The listing builds one solid part. Answer for the finished solid, in the listing's coordinates (mm). Face numbers are marked on the shaded views. A direction names the side the tool comes from. Round coordinates to 2 decimals unless told otherwise and drop trailing zeros. Order: outer loops, then holes, each group sorted by start corner. A loop starts at its lowest first (then second) coordinate and runs counter-clockwise, first axis right, second up. Notation, with made-up numbers: (38.5, -37) - (87.5, -37) arc R15 cw to (87.5, -18) - close; hole circle Ø8 at (10.5, 62). An arc over 180 degrees is marked (long way). Use CSV: the item, a comma, the result in double quotes. Start each with the question number.
Item 1: Straight lines are drawn through the part: line 1 along Y through (x, z) = (-11, 1.75); line 2 along Y through (x, z) = (-7, 3.95); line 3 along Y through (x, z) = (12, 0.8). For each, find the intervals that lie inside material, in ascending order. Write a range as [from, to].
Item 2: Find section A-A, the plane x = -5.5. Give the vertices of the cut face in (y, z).
Item 3: Find section D-D, the plane y = -3.5. Give the vertices of the cut face in (x, z), plus the area to 3 significant figures.
Item 4: Find section B-B, the plane z = 3.1. Count the separate pieces of the cut face and the enclosed holes in it, plus the area to 3 significant figures.
Item 5: For the marked faces 1 and 2, determine the directions among +Z, -Z, +X, -X, +Y, -Y from which every point of the face is accessible in a straight line to the end or side of a thin tool.
Item 6: Flat-ended cylindrical pins translate along their axes: P1, Ø3, axis at x = 11, y = 0, coming from the -Z side; P2, Ø2, axis at x = -5, z = 2, coming from the +Y side. Find the tip coordinate at first contact, or state that the pin passes through.
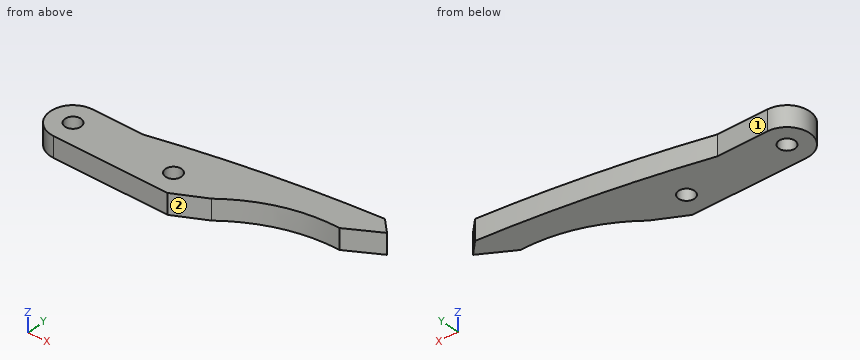
```python
from build123d import *

# Parameters (mm, degrees)
SKETCH1_R           = 5
SKETCH1_R_2         = 1.75
BOSS_EXTRUDE1_DEPTH = 4.5
BOSS_EXTRUDE2_START = -4.5
BOSS_EXTRUDE2_DEPTH = 4.5


with BuildPart() as part:
    # Sketch1 → Boss-Extrude1 (new body)
    # profile 1 of 3: a face of its own
    with BuildSketch(Plane.XY):
        with BuildLine():
            Line((11.000000016, 5), (-11, 5))
            ThreePointArc((-11, 5), (-7.464466094, 3.535533906), (-6, 0))
            ThreePointArc((-6, 0), (-7.464466094, -3.535533906), (-11, -5))
            Line((-11, -5), (11, -5))
            ThreePointArc((11, -5), (6, 8e-09), (11.000000016, 5))
        make_face()
    # profile 2 of 3: a face of its own
    with BuildSketch(Plane.XY):
        with Locations((-11, 0)):
            Circle(SKETCH1_R)
        with Locations((-11, 0)):
            Circle(SKETCH1_R_2, mode=Mode.SUBTRACT)
    # profile 3 of 3: a face of its own
    with BuildSketch(Plane.XY):
        with Locations((11, 0)):
            Circle(SKETCH1_R)
        with Locations((11, 0)):
            Circle(SKETCH1_R_2, mode=Mode.SUBTRACT)
    extrude(amount=BOSS_EXTRUDE1_DEPTH)

    # Sketch2 → Boss-Extrude2 (add)
    with BuildSketch(Plane.XY.offset(4.5).offset(BOSS_EXTRUDE2_START)):
        with BuildLine():
            Line((46.316479083, 12.87), (49.163214054, 10.06))
            Line((49.163214054, 10.06), (42.27, 6))
            add(Edge.make_bspline(
                [(42.27, 6), (30.146150748, 6.157348305), (20.61, -1.48)],
                knots=[0, 0, 0, 1, 1, 1], degree=2))
            Line((20.61, -1.48), (13.99, -5))
            Line((13.99, -5), (11, -5))
            ThreePointArc((11, -5), (16, 0), (11, 5))
            Line((11, 5), (0, 5))
            add(Edge.make_bspline(
                [(0, 5), (22.862881716, 10.69974244), (46.316479083, 12.87)],
                knots=[0, 0, 0, 1, 1, 1], degree=2))
        make_face()
    extrude(amount=BOSS_EXTRUDE2_DEPTH)


solid = part.part
```
Worked out:
1,line 1,"y = [-5, -1.75], [1.75, 5]"
1,line 2,"y = [-5, 5]"
1,line 3,"y = [-5, -1.44], [1.44, 7.74]"
2,outline,"(-5, 0) - (5, 0) - (5, 4.5) - (-5, 4.5) - close"
3,outline,"(-14.57, 0) - (16.81, 0) - (16.81, 4.5) - (-14.57, 4.5) - close"
3,area,"141 mm²"
4,separate pieces,"1"
4,enclosed holes,"2"
4,area,"560 mm²"
5,face 1,"+Z, -Z, -X, +Y"
5,face 2,"+Z, -Z, +X, -Y"
6,P1,"passes through"
6,P2,"stops at y = 5"
